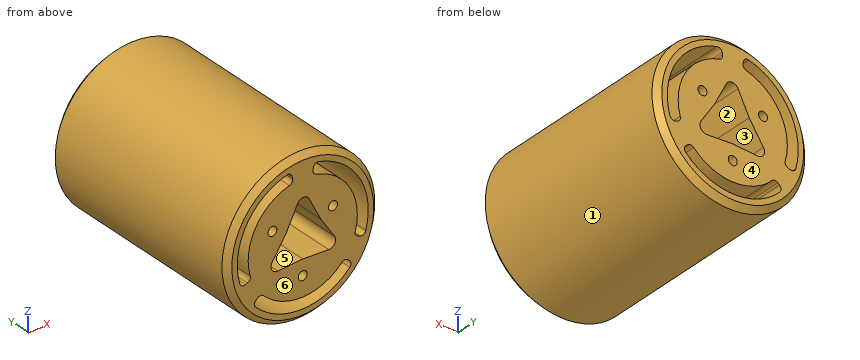
from build123d import *

# Parameters (mm, degrees)
SKETCH_1_R          = 35
EXTRUDE_1_DEPTH     = 100
SKETCH_2_R          = 2.05
CUT_EXTRUDE_1_DEPTH = 5
CHAMFER_1_SIZE      = 2.5
CUT_EXTRUDE_START   = -5
SKETCH_3_R          = 2.05
CUT_EXTRUDE_2_DEPTH = 5
CUT_EXTRUDE_3_DEPTH = 112.579568022


with BuildPart() as part:
    # ｽｹｯﾁ1 → ﾎﾞｽ - 押し出し1 (new body)
    with BuildSketch(Plane(origin=(0, 0, 0), x_dir=(1, 0, 0), z_dir=(0, 1, 0))):
        with Locations(Location((0, 0, 0), (0, 0, 270))):
            Circle(SKETCH_1_R)
    extrude(amount=EXTRUDE_1_DEPTH)

    # ｽｹｯﾁ2 → ｶｯﾄ - 押し出し1 (cut)
    with BuildSketch(Plane(origin=(0, 100, 0), x_dir=(1, 0, 0), z_dir=(0, 1, 0))):
        with Locations(Location((0, 16, 0), (0, 0, 270))):
            Circle(SKETCH_2_R)
        with Locations(Location((13.856406461, -8, 0), (0, 0, 270))):
            Circle(SKETCH_2_R)
        with Locations(Location((-13.856406461, -8, 0), (0, 0, 270))):
            Circle(SKETCH_2_R)
    extrude(amount=-CUT_EXTRUDE_1_DEPTH, mode=Mode.SUBTRACT)

    # 面取り1
    chamfer_1_edges = [part.edges().sort_by_distance(p)[0] for p in [
        (0, 0, -35),
        (0, 100, -35),
    ]]
    chamfer(chamfer_1_edges, length=CHAMFER_1_SIZE)

    # ｽｹｯﾁ3 → ｶｯﾄ - 押し出し2 (cut)
    with BuildSketch(Plane.XZ.offset(CUT_EXTRUDE_START)):
        with Locations(Location((0, -16, 0), (0, 0, 90))):
            Circle(SKETCH_3_R)
        with Locations(Location((-13.856406461, 8, 0), (0, 0, 90))):
            Circle(SKETCH_3_R)
        with Locations(Location((13.856406461, 8, 0), (0, 0, 90))):
            Circle(SKETCH_3_R)
    extrude(amount=CUT_EXTRUDE_2_DEPTH, mode=Mode.SUBTRACT)

    # ｽｹｯﾁ4 → ｶｯﾄ - 押し出し3 (cut, through all)
    with BuildSketch(Plane(origin=(0, 100, 0), x_dir=(1, 0, 0), z_dir=(0, 1, 0))):
        with BuildLine():
            Line((-21.394456976, 17.952080958), (-20.626377879, 17.307586071))
            ThreePointArc((-20.626377879, 17.307586071), (-19.240453869, 16.842194013), (-17.908150611, 17.444143479))
            ThreePointArc((-17.908150611, 17.444143479), (0, 25), (17.908150611, 17.444143479))
            ThreePointArc((17.908150611, 17.444143479), (19.240453869, 16.842194013), (20.626377879, 17.307586071))
            Line((20.626377879, 17.307586071), (21.394456976, 17.952080958))
            ThreePointArc((21.394456976, 17.952080958), (22.106227854, 19.38117195), (21.545230453, 20.875896261))
            ThreePointArc((21.545230453, 20.875896261), (0, 30), (-21.545230453, 20.875896261))
            ThreePointArc((-21.545230453, 20.875896261), (-22.106227854, 19.38117195), (-21.394456976, 17.952080958))
        make_face()
        with BuildLine():
            Line((4.849729672, -27.50418372), (4.675620276, -26.516760267))
            ThreePointArc((4.675620276, -26.516760267), (4.965540937, -25.083818837), (6.152996094, -24.230985103))
            ThreePointArc((6.152996094, -24.230985103), (21.650635095, -12.5), (24.061146705, 6.786841624))
            ThreePointArc((24.061146705, 6.786841624), (24.205994805, 8.241624824), (25.301998155, 9.209174196))
            Line((25.301998155, 9.209174196), (26.244186648, 9.552102762))
            ThreePointArc((26.244186648, 9.552102762), (27.837701191, 9.453968928), (28.851671716, 8.220768772))
            ThreePointArc((28.851671716, 8.220768772), (25.980762114, -15), (7.306441262, -29.096665034))
            ThreePointArc((7.306441262, -29.096665034), (5.731473337, -28.835140879), (4.849729672, -27.50418372))
        make_face()
        with BuildLine():
            Line((-26.244186648, 9.552102762), (-25.301998155, 9.209174196))
            ThreePointArc((-25.301998155, 9.209174196), (-24.205994805, 8.241624824), (-24.061146705, 6.786841624))
            ThreePointArc((-24.061146705, 6.786841624), (-21.650635095, -12.5), (-6.152996094, -24.230985103))
            ThreePointArc((-6.152996094, -24.230985103), (-4.965540937, -25.083818837), (-4.675620276, -26.516760267))
            Line((-4.675620276, -26.516760267), (-4.849729672, -27.50418372))
            ThreePointArc((-4.849729672, -27.50418372), (-5.731473337, -28.835140879), (-7.306441262, -29.096665034))
            ThreePointArc((-7.306441262, -29.096665034), (-25.980762114, -15), (-28.851671716, 8.220768772))
            ThreePointArc((-28.851671716, 8.220768772), (-27.837701191, 9.453968928), (-26.244186648, 9.552102762))
        make_face()
        with BuildLine():
            Line((-7.526031383, -4.935468734), (-14.052277383, 5.016317986))
            ThreePointArc((-14.052277383, 5.016317986), (-14.141048063, 8.162562133), (-11.37068313, 9.656486697))
            Line((-11.37068313, 9.656486697), (0, 9))
            Line((0, 9), (11.881623113, 9.676001467))
            ThreePointArc((11.881623113, 9.676001467), (14.65073581, 8.179757058), (14.559329968, 5.033588367))
            Line((14.559329968, 5.033588367), (8.305454246, -4.485468734))
            Line((8.305454246, -4.485468734), (2.950077133, -15.113256922))
            ThreePointArc((2.950077133, -15.113256922), (0.269735116, -16.763256659), (-2.409223974, -15.111012532))
            Line((-2.409223974, -15.111012532), (-7.526031383, -4.935468734))
        make_face()
    extrude(amount=-CUT_EXTRUDE_3_DEPTH, mode=Mode.SUBTRACT)


solid = part.part
Part model, mm, in its own coordinate system. Face numbers are marked on the shaded views. A direction names the side the tool comes from. Coordinates: 2 decimals unless noted, no trailing zeros. Loops run counter-clockwise (first coordinate to the right, second up) from the corner with the lowest first, then second, coordinate; pieces in that order, holes last. Notation, with made-up numbers: M -27,78.25 L 2,78.25 A27 ccw 2,115.25 Z; hole C 4,72 d4. An arc over 180 degrees is marked long. Use a Markdown table: item, result. Add a question column.
Q1. Pin check, flat tips, straight feed: P1, Ø3.5, axis at x = 0, z = -16, coming from the -Y side; P2, Ø10, axis at y = 16, z = 22.5, coming from the +X side; P3, Ø2, axis at y = 14, z = 13, coming from the +X side. Stop position of each tip, or through.
Q2. Cut at A-A (y = 74.5). Give the number of separate pieces and of enclosed holes in the cut face, and give its area (3 significant figures).
Q3. Mould opens along X. For the marked faces 1, 2, 3 and 4 say: +X half, -X half, draft (parallel to the pull), parting line (faces both ways), or undercut.
Q4. Cut at B-B (z = 0). Write the cut outline in (x, y).
Q5. Which spindle directions (+Z, -Z, +X, -X, +Y, -Y) get a long thin tool onto all of the face, cutting with end or side? Do the marked faces 5 and 6. Say none if no direction does.
Q6. Probe L1, parallel to X at y = 40, z = 13; L2, parallel to Z at x = 14.5, y = 60; L3, parallel to Z at x = 14, y = 71.5. List the from-to ranges inside material, lowest first.
Worked out:
| question | item | result |
|---|---|---|
| 1 | P1 | stops at y = 5 |
| 1 | P2 | stops at x = 30.31 |
| 1 | P3 | stops at x = 32.88 |
| 2 | separate pieces | 1 |
| 2 | enclosed holes | 4 |
| 2 | area | 2,680 mm2 |
| 3 | face 1 | parting line |
| 3 | face 2 | undercut |
| 3 | face 3 | undercut |
| 3 | face 4 | draft |
| 4 | outline | M -35,2.5 L -32.5,0 L -30,0 L -30,100 L -32.5,100 L -35,97.5 Z; M -25,0 L -10.76,0 L -10.76,100 L -25,100 Z; M 11.25,0 L 25,0 L 25,100 L 11.25,100 Z; M 30,0 L 32.5,0 L 35,2.5 L 35,97.5 L 32.5,100 L 30,100 Z |
| 5 | face 5 | +Y, -Y |
| 5 | face 6 | +Z, -Z, +X, -X, -Y |
| 6 | L1 | x = -32.5 to -27.04, -21.35 to -3.47, 4.01 to 21.35, 27.04 to 32.5 |
| 6 | L2 | z = -31.86 to -26.26, -20.37 to -8.42, -4.94 to 20.37, 26.26 to 31.86 |
| 6 | L3 | z = -32.08 to -26.53, -20.71 to -8.96, -4.18 to 20.71, 26.53 to 32.08 |
